Autodesk Fusion 360 part; units mm, degrees
sketch "スケッチ1" plane through (0, 0, 0) normal (0, 0, 1) x (1, 0, 0) in component "Component"
  line L0 (-3.4641, 12.5) -> (-1.7321, 9.5)
  line L1 (-1.7321, 9.5) -> (1.7321, 9.5)
  line L2 (1.7321, 9.5) -> (3.4641, 12.5)
  line L3 (3.4641, 12.5) -> (1.7321, 15.5)
  line L4 (1.7321, 15.5) -> (-1.7321, 15.5)
  line L5 (-1.7321, 15.5) -> (-3.4641, 12.5)
  line L6 (0, 150) -> (0, -150) construction
  line L7 (-100, 0) -> (234.7346, 0) construction
  line L8 (-3.4641, -12.5) -> (-1.7321, -9.5)
  line L9 (-1.7321, -9.5) -> (1.7321, -9.5)
  line L10 (3.4641, -12.5) -> (1.7321, -15.5)
  line L11 (-1.7321, -15.5) -> (-3.4641, -12.5)
  line L12 (1.7321, -9.5) -> (3.4641, -12.5)
  line L13 (1.7321, -15.5) -> (-1.7321, -15.5)
  line L14 (-31, 8) -> (50, 8)
  line L15 (-3.4641, 12.5) -> (-3.4641, 34)
  line L16 (-3.4641, 34) -> (3.4641, 34)
  line L17 (3.4641, 34) -> (3.4641, -18)
  line L18 (3.4641, -18) -> (-3.4641, -18)
  line L19 (-3.4641, -18) -> (-3.4641, 12.5)
  line L20 (-3.4641, 34) -> (-3.4641, 36.5)
  line L21 (-3.4641, 36.5) -> (3.4641, 36.5)
  line L22 (3.4641, 36.5) -> (3.4641, 34)
  line L23 (-3.4641, -18) -> (-3.4641, -20.5)
  line L24 (-3.4641, -20.5) -> (3.4641, -20.5)
  line L25 (3.4641, -20.5) -> (3.4641, -18)
  line L26 (3.4641, 11.4641) -> (31, 11.4641)
  line L27 (31, 11.4641) -> (31, 4.5359)
  line L28 (31, 4.5359) -> (3.4641, 4.5359)
  line L29 (31, 11.4641) -> (33.5, 11.4641)
  line L30 (33.5, 11.4641) -> (33.5, 4.5359)
  line L31 (33.5, 4.5359) -> (31, 4.5359)
  point P0 (0, 12.5)
  point P1 (0, -12.5)
  dimension "d1" = 6
  dimension "d2" = 25
  dimension "d3" = 8
  dimension "d4" = 52
  dimension "d5" = 2.5
  dimension "d6" = 2.5
  dimension "d7" = 31
extrude "押し出し1" add sketch "スケッチ1" against normal blind 2.5 contours L0 L1 L2 L3 L4 L5 | L8 L9 L10 L11 L12 L13 makes body 1 at (-0.5774, 11.5, 0) makes body 2 at (-0.5774, -11.5, 0) in component "Component"
extrude "押し出し2" add sketch "スケッチ1" along normal blind 2.5 contours L0 L1 L2 L3 L4 L5 | L3 L4 L5 L15 L16 L17 | L0 L1 L2 L14 L17 L19 | L8 L9 L12 L14 L17 L19 | L14 L17 L26 L27 | L14 L17 L27 L28 | L8 L9 L10 L11 L12 L13 | L10 L11 L13 L17 L18 L19 bodies 1 2 in component "Component"
extrude "押し出し3" add sketch "スケッチ1" along normal blind 14 contours L16 L20 L21 L22 | L14 L27 L29 L30 | L14 L27 L30 L31 | L18 L23 L24 L25 bodies 1 in component "Component"
sketch "スケッチ2" plane through (0, 0, 2.5) normal (0, 0, 1) x (-1, 0, 0) in component "Component"
  line L0 (-31, -4.5359) -> (-31, -11.4641)
  line L1 (-31, -11.4641) -> (-3.4641, -11.4641)
  line L2 (-3.4641, -11.4641) -> (-3.4641, -34)
  line L3 (-3.4641, -34) -> (3.4641, -34)
  line L4 (3.4641, -34) -> (3.4641, 18)
  line L5 (3.4641, 18) -> (-3.4641, 18)
  line L6 (-3.4641, 18) -> (-3.4641, -4.5359)
  line L7 (-3.4641, -4.5359) -> (-31, -4.5359)
  circle A0 centre (0, -12.5) radius 1.5
  circle A1 centre (0, 12.5) radius 1.5
  point P0 (0, -12.5)
  point P1 (0, 12.5)
  dimension "d14" = 3
hole "穴1" at (0, 12.5, 2.5) at (0, -12.5, 2.5) direction (0, 0, -1) diameter 3 depth 10 tip angle 118 countersink diameter 6 countersink angle 90 bodies 1 in component "Component"
fillet "フィレット1" radius 2.5 4 edges at (3.4641, 35.25, 14) (3.4641, -19.25, 14) (32.25, 4.5359, 14) (32.25, 11.4641, 14) on bodies 1 in component "Component"
component "Component" placed x (1, 0, 0) y (0, 1, 0) z (0, 0, 1) at (0, 0, 0)
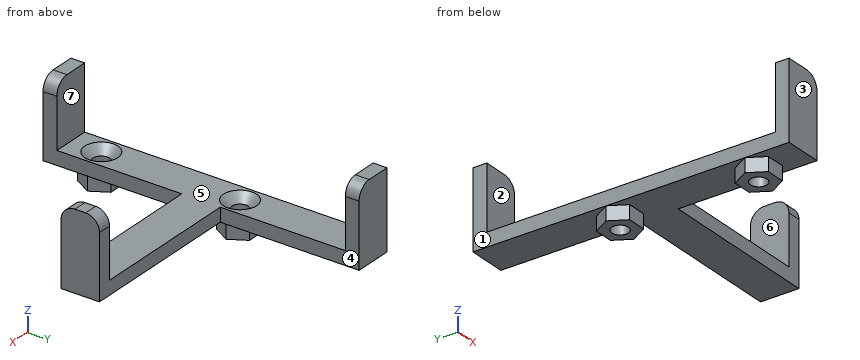
The model under review builds one solid part; all positions refer to its coordinate system, in mm. Face numbers are marked on the shaded views. A direction names the side the tool comes from. Give positions to 0.01 mm unless a question says otherwise; leave off trailing zeros. Loops run counter-clockwise (first coordinate to the right, second up) from the corner with the lowest first, then second, coordinate; pieces in that order, holes last. Notation, with made-up numbers: (59.25, -13.5) -> (118.25, -13.5) arc R8 cw to (118.25, 1.5) -> close; hole circle Ø7 at (-34.5, -28). An arc over 180 degrees is marked (long way). Write each question's results on one line, items separated by ' | '.
1) Take a section at B-B, the plane z = 8.75. Give the boundary of the cut face in (x, y), plus the area to 3 significant figures.
Conclusion:
outline: (-3.46, -20.5) -> (3.46, -20.5) -> (3.46, -18) -> (-3.46, -18) -> close; (-3.46, 34) -> (3.46, 34) -> (3.46, 36.5) -> (-3.46, 36.5) -> close; (31, 4.54) -> (33.5, 4.54) -> (33.5, 11.46) -> (31, 11.46) -> close | area: 52.0 mm^2
2) Take a section at A-A, the plane x = 0. Give the boundary of the cut face in (y, z).
Conclusion:
outline: (-20.5, 0) -> (-15.5, 0) -> (-15.5, -2.5) -> (-14, -2.5) -> (-14, 1) -> (-15.5, 2.5) -> (-18, 2.5) -> (-18, 14) -> (-20.5, 14) -> close; (-11, -2.5) -> (-9.5, -2.5) -> (-9.5, 0) -> (9.5, 0) -> (9.5, -2.5) -> (11, -2.5) -> (11, 1) -> (9.5, 2.5) -> (-9.5, 2.5) -> (-11, 1) -> close; (14, -2.5) -> (15.5, -2.5) -> (15.5, 0) -> (36.5, 0) -> (36.5, 14) -> (34, 14) -> (34, 2.5) -> (15.5, 2.5) -> (14, 1) -> close
3) For line 1 along Y through (x, z) = (3, 11.25); line 2 along X through (y, z) = (12.5, -1); line 3 along Y through (x, z) = (0, -1.1), list the stretches that pass through material, from the lowest coordinate up. Write a range as from..to.
Conclusion:
line 1: y = -20.5..-18, 34..36.5 | line 2: x = -3.46..-1.5, 1.5..3.46 | line 3: y = -15.5..-14, -11..-9.5, 9.5..11, 14..15.5
4) Insertion check: pin 1 Ø2 at (x, z) = (4, 3.5) entering from -Y; pin 2 Ø12 at (x, y) = (29, 7) entering from -Z; pin 3 Ø0.8 at (x, z) = (-0.5, -1) entering from -Y; pin 4 Ø3 at (x, z) = (0.5, -2) entering from +Y. Each pin has a flat end and moves straight along its axis. Give the tip position at first contact, or say it passes through.
Conclusion:
pin 1: stops at y = -20.5 | pin 2: stops at z = 0 | pin 3: stops at y = -15.5 | pin 4: stops at y = 15.5
5) Tool access review of the marked faces 4, 5, 6 and 7: name each direction out of +Z, -Z, +X, -X, +Y, -Y from which nothing blocks a thin tool from reaching the whole face with its end or side.
Conclusion:
face 4: +Z, -Z, +X, +Y | face 5: +Z, -X | face 6: +Z, -X, +Y, -Y | face 7: +Z, +X, -X
6) Take a section at D-D, the plane x = 13.5. Give the boundary of the cut face in (y, z), plus the area to 3 significant figures.
Conclusion:
outline: (4.54, 0) -> (11.46, 0) -> (11.46, 2.5) -> (4.54, 2.5) -> close | area: 17.3 mm^2
7) Draft analysis for pull direction Y (two halves, no side actions). For the marked faces 1, 2 and 3, state which applies: pulls with the +Y half, pulls with the -Y half, needs draft (parallel to the pull), parting line crosses it, or undercut.
Conclusion:
face 1: needs draft | face 2: undercut | face 3: pulls with the -Y half
8) Take a section at C-C, the plane y = 32.5. Give the boundary of the cut face in (x, z).
Conclusion:
outline: (-3.46, 0) -> (3.46, 0) -> (3.46, 2.5) -> (-3.46, 2.5) -> close
